```python
from build123d import *

# Parameters (mm, degrees)
SKETCH1_R           = 37
BOSS_EXTRUDE1_DEPTH = 1
SKETCH2_R           = 1.5
BOSS_EXTRUDE2_DEPTH = 3
SKETCH16_R          = 1.5
CUT_EXTRUDE9_DEPTH  = 5
CIRPATTERN1_COUNT   = 3
SKETCH5_R           = 75.500139874
CUT_EXTRUDE3_DEPTH  = 2
CIRPATTERN2_COUNT   = 3
FILLET2_R           = 1
SKETCH18_R          = 1
CUT_EXTRUDE10_DEPTH = 2
SKETCH20_W          = 22
SKETCH20_H          = 10
CUT_EXTRUDE12_DEPTH = 2
FILLET3_R           = 4


with BuildPart() as part:
    # Sketch1 → Boss-Extrude1 (new body)
    with BuildSketch(Plane(origin=(0, 0, 0), x_dir=(1, 0, 0), z_dir=(0, 1, 0))):
        Circle(SKETCH1_R)
    extrude(amount=BOSS_EXTRUDE1_DEPTH)

    # Sketch2 → Boss-Extrude2 (add)
    with BuildSketch(Plane(origin=(0, 1, 0), x_dir=(1, 0, 0), z_dir=(0, 1, 0))):
        with BuildLine():
            Line((-12.654745303, 34.768626969), (-9.918584156, 27.251086003))
            ThreePointArc((-9.918584156, 27.251086003), (0, 29), (9.918584156, 27.251086003))
            Line((9.918584156, 27.251086003), (12.654745303, 34.768626969))
            ThreePointArc((12.654745303, 34.768626969), (0, 37), (-12.654745303, 34.768626969))
        make_face()
        with Locations((0, 32)):
            Circle(SKETCH2_R, mode=Mode.SUBTRACT)
    boss_extrude2 = extrude(amount=BOSS_EXTRUDE2_DEPTH)

    # Sketch16 → Cut-Extrude9 (cut, through all)
    with BuildSketch(Plane(origin=(0, 4, 0), x_dir=(1, 0, 0), z_dir=(0, 1, 0))):
        with Locations((0, 32)):
            Circle(SKETCH16_R)
    cut_extrude9 = extrude(amount=-CUT_EXTRUDE9_DEPTH, mode=Mode.SUBTRACT)

    # CirPattern1: Boss-Extrude2, Cut-Extrude9 ×3 about axis
    cirpattern1_axis = Axis((0, 0, 0), (0, 1, 0))
    for i in range(1, CIRPATTERN1_COUNT):
        add(boss_extrude2.rotate(cirpattern1_axis, i * 360 / CIRPATTERN1_COUNT))
        add(cut_extrude9.rotate(cirpattern1_axis, i * 360 / CIRPATTERN1_COUNT), mode=Mode.SUBTRACT)

    # Sketch5 → Cut-Extrude3 (cut, through all)
    with BuildSketch(Plane(origin=(0, 1, 0), x_dir=(1, 0, 0), z_dir=(0, 1, 0))):
        with Locations((86.602540378, 50)):
            Circle(SKETCH5_R)
    cut_extrude3 = extrude(amount=-CUT_EXTRUDE3_DEPTH, mode=Mode.SUBTRACT)

    # CirPattern2: Cut-Extrude3 ×3 about axis
    cirpattern2_axis = Axis((0, 0, 0), (0, 1, 0))
    for i in range(1, CIRPATTERN2_COUNT):
        add(cut_extrude3.rotate(cirpattern2_axis, i * 360 / CIRPATTERN2_COUNT), mode=Mode.SUBTRACT)

    # Fillet2
    fillet2_edges = [part.edges().sort_by_distance(p)[0] for p in [
        (-9.918584156, 2.5, -27.251086003),
        (9.918584156, 2.5, -27.251086003),
        (-18.640840681, 2.5, 22.21528885),
        (-28.559424837, 2.5, 5.035797152),
        (28.559424837, 2.5, 5.035797152),
        (18.640840681, 2.5, 22.21528885),
    ]]
    fillet(fillet2_edges, radius=FILLET2_R)

    # Sketch18 → Cut-Extrude10 (cut, through all)
    with BuildSketch(Plane(origin=(0, 1, 0), x_dir=(1, 0, 0), z_dir=(0, 1, 0))):
        with Locations((9, 5.5)):
            Circle(SKETCH18_R)
        with Locations((-9, 5.5)):
            Circle(SKETCH18_R)
        with Locations((9, -5.5)):
            Circle(SKETCH18_R)
        with Locations((-9, -5.5)):
            Circle(SKETCH18_R)
    extrude(amount=-CUT_EXTRUDE10_DEPTH, mode=Mode.SUBTRACT)

    # Sketch20 → Cut-Extrude12 (cut, through all)
    with BuildSketch(Plane(origin=(0, 1, 0), x_dir=(1, 0, 0), z_dir=(0, 1, 0))):
        with Locations((0, -17.5)):
            Rectangle(SKETCH20_W, SKETCH20_H)
    extrude(amount=-CUT_EXTRUDE12_DEPTH, mode=Mode.SUBTRACT)

    # Fillet3
    fillet3_edges = [part.edges().sort_by_distance(p)[0] for p in [
        (11, 0.5, 12.5),
        (11, 0.5, 22.5),
        (-11, 0.5, 22.5),
        (-11, 0.5, 12.5),
    ]]
    fillet(fillet3_edges, radius=FILLET3_R)


solid = part.part
```
For this review, take the finished solid that the model builds, in its own axes (mm). A direction names the side the tool comes from. Round coordinates to 2 decimals unless told otherwise and drop trailing zeros. Write each loop counter-clockwise with the first axis right and the second up, starting at its lowest first coordinate (ties: lowest second). Pieces come first, ordered by that corner, then holes. Notation, with made-up numbers: M 1,82 L 49,82 A22 cw 49,101 Z; hole C 38,-11 d2. An arc over 180 degrees is marked long. One line per item, written item: value. Start each with the question number.
(1) We need section B-B (z = -32). Give the boundary of the cut face in (x, y), and give its area (3 significant figures).
(2) Machinability: for faces 1 (the flat face through (33.031, 2.479, 5.824)), 2 (the flat face through (-21.56, 2.479, 25.694)), 3 (the cylindrical face through (9.859, 0.493, 13.703)), 4 (the cylindrical face through (-25.05, 2.48, 14.61)), which of the approach directions +Z, -Z, +X, -X, +Y, -Y give a long, thin tool a straight path to every point of the face, cutting with its end or side? Answer none if there is none.
(3) Insertion check: pin 1 (2 mm diameter, centred on x = 1.5, z = -13.5, fed in from +Y); pin 2 (1.1 mm diameter, centred on x = 1.5, y = 0.5, fed in from -Z); pin 3 (0.8 mm diameter, centred on y = 0.5, z = 17.5, fed in from +X). Each pin has a flat end and moves straight along its axis. Give the tip position at first contact, or say it passes through.
(4) We need section C-C (y = 1.7). Give the boundary of the cut face in (x, z).
(5) We need section D-D (z = -5.5). Give the boundary of the cut face in (x, y).
(6) The part is to be moulded in two halves that separate along X. For faces 5 (the flat face through (-11.472, 2.479, -31.518)), 6 (the cylindrical face through (-9.797, 0.493, 21.359)), 7 (the flat face through (-30, 4, 17)), say which applies: released by +X, released by -X, zero draft, split by the parting line, or undercut.
(7) We need section A-A (x = 0). Give the boundary of the cut face in (y, z).
(8) Wall thickness on line 1 (X direction, y = 3.85, z = 17); line 2 (Z direction, x = 9, y = 0.45); line 3 (Y direction, x = 11.5, z = 24): over which ranges is each line inside the solid? List them lowest first.
Result:
1. outline: M -13.28,0 L -1.5,0 L -1.5,4 L -11.65,4 L -11.65,1 L -13.28,1 Z; M 1.5,0 L 13.28,0 L 13.28,1 L 11.65,1 L 11.65,4 L 1.5,4 Z
1. area: 84.4 mm²
2. face 1: -Z, +X, +Y
2. face 2: +Z, +Y
2. face 3: +Y, -Y
2. face 4: -Z, +Y
3. pin 1: y = 1
3. pin 2: z = -36.99
3. pin 3: x = 32.81
4. outline: M -36.44,6.42 L -29.53,5.21 A1 ccw -28.38,5.98 A29 cw -19.37,21.58 A1 ccw -19.27,22.97 L -23.78,28.34 A37 ccw Z; M -12.65,-34.77 A37 ccw 12.65,-34.77 L 10.25,-28.18 A1 ccw 9,-27.57 A29 cw -9,-27.57 A1 ccw -10.25,-28.18 Z; M 19.27,22.97 A1 ccw 19.37,21.58 A29 cw 28.38,5.98 A1 ccw 29.53,5.21 L 36.44,6.42 A37 ccw 23.78,28.34 Z; hole C -27.71,16 d3; hole C 0,-32 d3; hole C 27.71,16 d3
5. outline: M -25.61,0 L -10,0 L -10,1 L -25.61,1 Z; M -8,0 L 8,0 L 8,1 L -8,1 Z; M 10,0 L 25.61,0 L 25.61,1 L 10,1 Z
6. face 5: released by -X
6. face 6: undercut
6. face 7: zero draft
7. outline: M 0,-37 L 4,-37 L 4,-33.5 L 0,-33.5 Z; M 0,-30.5 L 4,-30.5 L 4,-29 L 1,-29 L 1,12.5 L 0,12.5 Z; M 0,22.5 L 1,22.5 L 1,24.5 L 0,24.5 Z
8. line 1: -32.86 to -28.83, -26.59 to -23.49, 23.49 to 26.59, 28.83 to 32.86
8. line 2: -35.89 to -6.5, -4.5 to 4.5, 6.5 to 13.04, 21.96 to 25.04
8. line 3: 0 to 1
